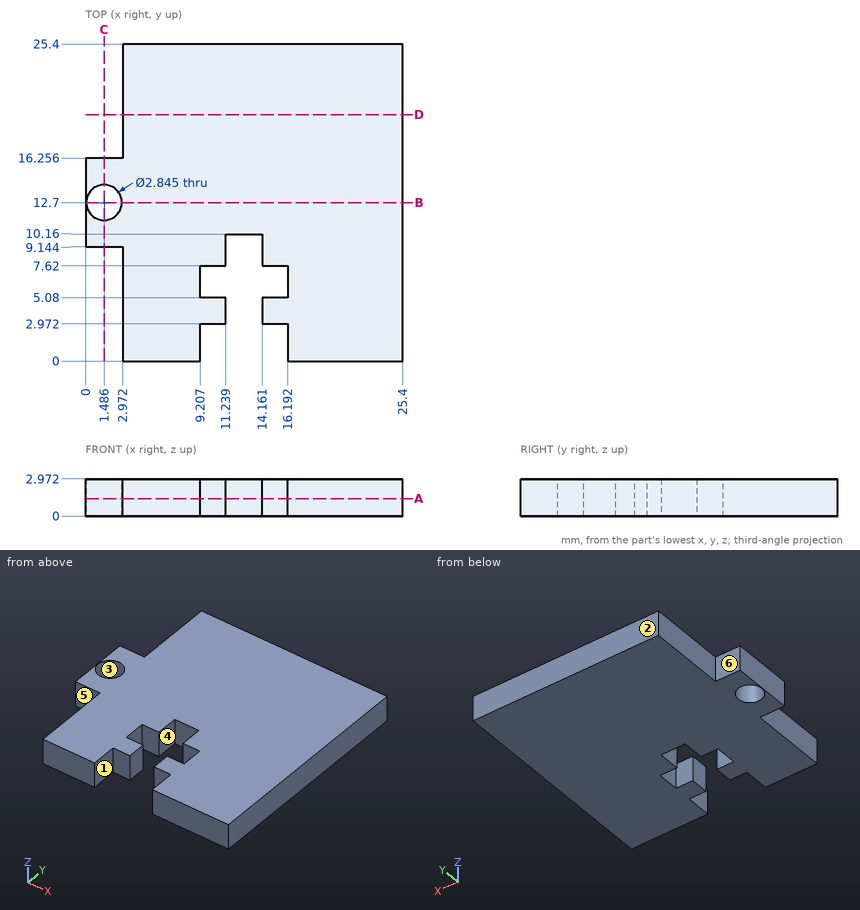
Can you work these out from the drawing? Everything is in mm from the part's minimum corner. A direction names the side the tool comes from. Coordinates: 2 decimals unless noted, no trailing zeros. Order: outer loops, then holes, each group sorted by start corner. A loop starts at its lowest first (then second) coordinate and runs counter-clockwise, first axis right, second up. Notation, with made-up numbers: (80.25, 61.25) -> (101.25, 61.25) arc R26 ccw to (101.25, 96.25) -> close; hole circle Ø10 at (17.25, -18). An arc over 180 degrees is marked (long way). Use one line per item in the form item = value.
Q1. I need wall thicknesses on L1, parallel to Y at x = 9.25, z = 1.4; L2, parallel to X at y = 1.75, z = 2.5; L3, parallel to X at y = 3.5, z = 1.1. Which ranges of each line are inside material? Lowest first, please.
From the geometry:
L1 = 2.97 to 5.08, 7.62 to 25.4
L2 = 2.97 to 9.21, 16.19 to 25.4
L3 = 2.97 to 11.24, 14.16 to 25.4
Q2. We'd pull the mould along Y, two halves only. Please class the marked faces 1, 2 and 3: released by +Y, released by -Y, zero draft, split by the parting line, or undercut.
From the geometry:
face_1 = zero draft
face_2 = released by +Y
face_3 = undercut
Q3. Imagine slicing it at C-C, the plane x = 1.5. List the corners of the cut face in (y, z) for me (1 decimal).
From the geometry:
outline = (9.1, 0) -> (11.3, 0) -> (11.3, 3) -> (9.1, 3) -> close; (14.1, 0) -> (16.3, 0) -> (16.3, 3) -> (14.1, 3) -> close
Q4. Which directions (+Z, -Z, +X, -X, +Y, -Y) give clear straight access to the entire face, cutting with the end or side of a thin tool? Please do the marked faces 4, 5 and 6.
From the geometry:
face_4 = +Z, -Z, -Y
face_5 = +Z, -Z, -X, -Y
face_6 = +Z, -Z, -X, +Y
Q5. Imagine slicing it at A-A, the plane z = 1.4. List the corners of the cut face in (x, y) for me (1 decimal).
From the geometry:
outline = (0, 9.1) -> (3, 9.1) -> (3, 0) -> (9.2, 0) -> (9.2, 3) -> (11.2, 3) -> (11.2, 5.1) -> (9.2, 5.1) -> (9.2, 7.6) -> (11.2, 7.6) -> (11.2, 10.2) -> (14.2, 10.2) -> (14.2, 7.6) -> (16.2, 7.6) -> (16.2, 5.1) -> (14.2, 5.1) -> (14.2, 3) -> (16.2, 3) -> (16.2, 0) -> (25.4, 0) -> (25.4, 25.4) -> (3, 25.4) -> (3, 16.3) -> (0, 16.3) -> close; hole circle Ø2.8 at (1.5, 12.7)
Q6. Will these pins go through, and if not, where does the flat tip stop? P1, Ø1.5, axis at x = 1.5, z = 1, coming from the -Y side; P2, Ø0.6, axis at x = 10.5, z = 2, coming from the -Y side.
From the geometry:
P1 = 9.14
P2 = 2.97
Q7. Imagine slicing it at D-D, the plane y = 19.75. List the corners of the cut face in (x, z) for me.
From the geometry:
outline = (2.97, 0) -> (25.4, 0) -> (25.4, 2.97) -> (2.97, 2.97) -> close
Q8. Imagine slicing it at B-B, the plane y = 12.7. List the corners of the cut face in (x, z) for me.
From the geometry:
outline = (0, 0) -> (0.06, 0) -> (0.06, 2.97) -> (0, 2.97) -> close; (2.91, 0) -> (25.4, 0) -> (25.4, 2.97) -> (2.91, 2.97) -> close
